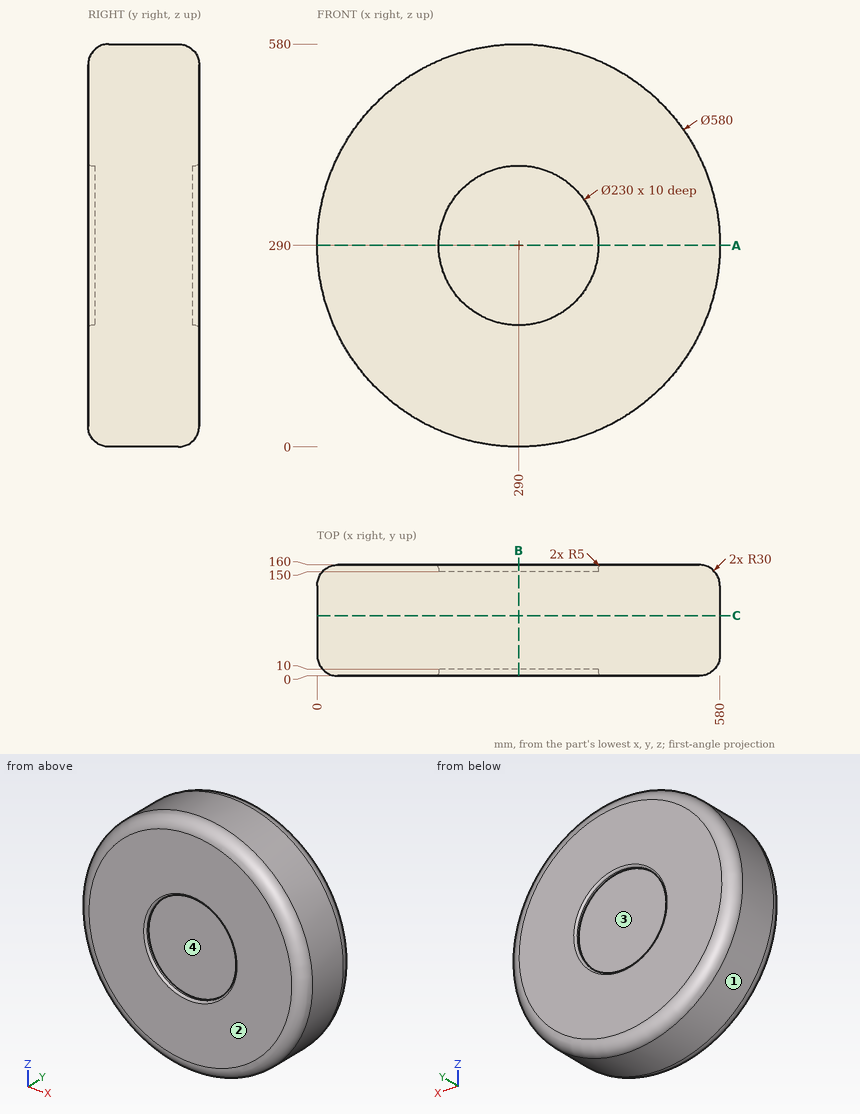
Verification items for this drawing (mm, ordinates from the low corner). Coordinates: 2 decimals unless noted, no trailing zeros. Order: outer loops, then holes, each group sorted by start corner. A loop starts at its lowest first (then second) coordinate and runs counter-clockwise, first axis right, second up. Notation, with made-up numbers: M 31,47.5 L 62,47.5 A11 cw 62,60.5 Z; hole C 87,47 d7. An arc over 180 degrees is marked long. Use CSV: the item, a comma, the result in double quotes.
Item 1: Mould release check, pull along Z, two halves, no side actions. Record for the marked faces 1, 2, 3 and 4: pulls with the +Z half, pulls with the -Z half, needs draft (parallel to the pull), parting line crosses it, or undercut.
Returned:
face 1,"parting line crosses it"
face 2,"needs draft"
face 3,"undercut"
face 4,"undercut"
Item 2: Thickness scan on line 1 along X through (y, z) = (7, 290); line 2 along X through (y, z) = (8.8, 290); line 3 along Y through (x, z) = (31, 251). Record the ranges inside material, lowest first.
Returned:
line 1,"x = 10.74 to 175, 405 to 569.26"
line 2,"x = 8.77 to 175, 405 to 571.23"
line 3,"y = 0.06 to 159.94"
Item 3: Cross-section at C-C on y = 87. Record the cut outline in (x, z).
Returned:
outline,"C 290,290 d580"
Item 4: Gauge pin test, flat ends, axial feed: pin 1 Ø12 at (y, z) = (82, 104.5) entering from +X; pin 2 Ø3 at (y, z) = (42.5, 430) entering from +X; pin 3 Ø4 at (x, y) = (76, 54.5) entering from +Z; pin 4 Ø8 at (x, z) = (409, 279) entering from -Y. Record the tip position at first contact, or that the pin passes through.
Returned:
pin 1,"stops at x = 517.77"
pin 2,"stops at x = 544.79"
pin 3,"stops at z = 487.88"
pin 4,"stops at y = 0"
Item 5: Cross-section at B-B on x = 290. Record the cut outline in (y, z), then the cut area to 3 significant figures.
Returned:
outline,"M 0,30 A30 ccw 30,0 L 130,0 A30 ccw 160,30 L 160,170 A5 ccw 155,175 L 150,175 L 150,405 L 155,405 A5 ccw 160,410 L 160,550 A30 ccw 130,580 L 30,580 A30 ccw 0,550 L 0,410 A5 ccw 5,405 L 10,405 L 10,175 L 5,175 A5 ccw 0,170 Z"
area,"87,400 mm2"
Item 6: Cross-section at A-A on z = 290. Record the cut outline in (x, y).
Returned:
outline,"M 0,30 A30 ccw 30,0 L 170,0 A5 ccw 175,5 L 175,10 L 405,10 L 405,5 A5 ccw 410,0 L 550,0 A30 ccw 580,30 L 580,130 A30 ccw 550,160 L 410,160 A5 ccw 405,155 L 405,150 L 175,150 L 175,155 A5 ccw 170,160 L 30,160 A30 ccw 0,130 Z"
